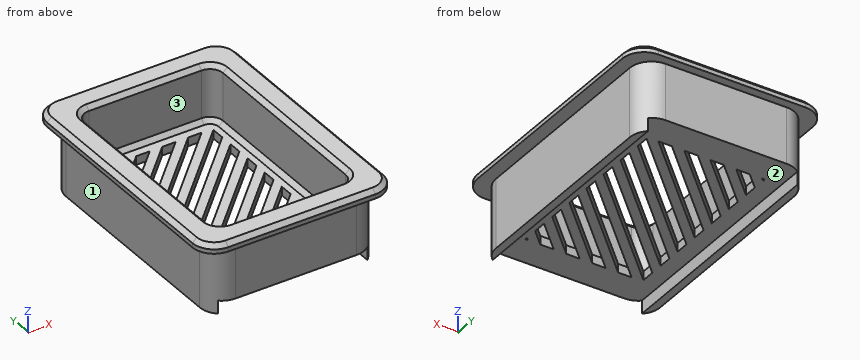
```python
from build123d import *

# Parameters (mm, degrees)
F0_W      = 28
F0_H      = 44
F1_DEPTH  = 2
F3_DEPTH  = 2
F4_W      = 38
F4_H      = 57
F4_W_2    = 27
F4_H_2    = 43
F5_DEPTH  = 2
F6_W      = 1.75
F6_H      = 57
F7_DEPTH  = 3
F8_W      = 38
F8_H      = 57
F8_W_2    = 32
F8_H_2    = 49
F9_DEPTH  = 11
F10_W     = 44
F10_H     = 61
F10_W_2   = 32
F10_H_2   = 49
F11_DEPTH = 2
F12_R     = 5
F13_R     = 3
F14_SIZE  = 1


with BuildPart() as f1:
    # F0 (on Top) → F1 (new body)
    with BuildSketch(Plane.XY):
        with Locations((-14, 22)):
            Rectangle(F0_W, F0_H)
    extrude(amount=F1_DEPTH)

    # F2 (on face) → F3 (cut, through all)
    with BuildSketch(Plane.XY.offset(2)):
        Polygon((-28, 48.4443650814), (-1.0000491969, 75.4443158845), (0, 79.5556349186), (-29.5556349186, 50), align=None)
        Polygon((0, 79.5556349186), (-1.0000491969, 75.4443158845), (1.5556349186, 78), align=None)
        Polygon((-28, 42.4443650814), (-2.9286171114, 67.51574797), (-1.9285679145, 71.6270670041), (-29.5556349186, 44), align=None)
        Polygon((-1.9285679145, 71.6270670041), (-2.9286171114, 67.51574797), (1.5556349186, 72), (0, 73.5556349186), align=None)
        Polygon((-28, 36.4443650814), (-4.8571850259, 59.5871800555), (-3.857135829, 63.6984990896), (-29.5556349186, 38), align=None)
        Polygon((-3.857135829, 63.6984990896), (-4.8571850259, 59.5871800555), (1.5556349186, 66), (0, 67.5556349186), align=None)
        Polygon((-28, 30.4443650814), (-6.7857529404, 51.658612141), (-5.7857037435, 55.7699311751), (-29.5556349186, 32), align=None)
        Polygon((-5.7857037435, 55.7699311751), (-6.7857529404, 51.658612141), (1.5556349186, 60), (0, 61.5556349186), align=None)
        Polygon((-28, 24.4443650814), (-8.7143208549, 43.7300442265), (-7.714271658, 47.8413632606), (-29.5556349186, 26), align=None)
        Polygon((-7.714271658, 47.8413632606), (-8.7143208549, 43.7300442265), (1.5556349186, 54), (0, 55.5556349186), align=None)
        Polygon((-28, 18.4443650814), (-10.6428887694, 35.8014763119), (-9.6428395725, 39.9127953461), (-29.5556349186, 20), align=None)
        Polygon((-9.6428395725, 39.9127953461), (-10.6428887694, 35.8014763119), (1.5556349186, 48), (0, 49.5556349186), align=None)
        Polygon((-28, 12.4443650814), (-12.5714566839, 27.8729083974), (-11.571407487, 31.9842274316), (-29.5556349186, 14), align=None)
        Polygon((-11.571407487, 31.9842274316), (-12.5714566839, 27.8729083974), (1.5556349186, 42), (0, 43.5556349186), align=None)
        Polygon((-28, 6.4443650814), (-14.5000245985, 19.9443404829), (-13.4999754015, 24.0556595171), (-29.5556349186, 8), align=None)
        Polygon((-13.4999754015, 24.0556595171), (-14.5000245985, 19.9443404829), (1.5556349186, 36), (0, 37.5556349186), align=None)
        Polygon((-28, 0.4443650814), (-16.428592513, 12.0157725684), (-15.4285433161, 16.1270916026), (-29.5556349186, 2), align=None)
        Polygon((-15.4285433161, 16.1270916026), (-16.428592513, 12.0157725684), (1.5556349186, 30), (0, 31.5556349186), align=None)
        Polygon((-28, -5.5556349186), (-18.3571604275, 4.0872046539), (-17.3571112306, 8.1985236881), (-29.5556349186, -4), align=None)
        Polygon((-17.3571112306, 8.1985236881), (-18.3571604275, 4.0872046539), (1.5556349186, 24), (0, 25.5556349186), align=None)
        Polygon((-28, -11.5556349186), (-20.285728342, -3.8413632606), (-19.2856791451, 0.2699557735), (-29.5556349186, -10), align=None)
        Polygon((-19.2856791451, 0.2699557735), (-20.285728342, -3.8413632606), (1.5556349186, 18), (0, 19.5556349186), align=None)
        Polygon((-28, -17.5556349186), (-22.2142962565, -11.7699311751), (-21.2142470596, -7.658612141), (-29.5556349186, -16), align=None)
        Polygon((-21.2142470596, -7.658612141), (-22.2142962565, -11.7699311751), (1.5556349186, 12), (0, 13.5556349186), align=None)
        Polygon((-28, -23.5556349186), (-24.142864171, -19.6984990896), (-23.1428149741, -15.5871800555), (-29.5556349186, -22), align=None)
        Polygon((-23.1428149741, -15.5871800555), (-24.142864171, -19.6984990896), (1.5556349186, 6), (0, 7.5556349186), align=None)
        Polygon((-28, -29.5556349186), (-26.0714320855, -27.6270670041), (-25.0713828886, -23.51574797), (-29.5556349186, -28), align=None)
        Polygon((-25.0713828886, -23.51574797), (-26.0714320855, -27.6270670041), (1.5556349186, 0), (0, 1.5556349186), align=None)
        Polygon((-26.9999508031, -31.4443158845), (-29.5556349186, -34), (-28, -35.5556349186), align=None)
        Polygon((0, -4.4443650814), (-26.9999508031, -31.4443158845), (-28, -35.5556349186), (1.5556349186, -6), align=None)
    extrude(amount=-F3_DEPTH, mode=Mode.SUBTRACT)

    # F4 (on Top) → F5 (join)
    with BuildSketch(Plane.XY):
        with Locations((-14, 22)):
            Rectangle(F4_W, F4_H)
        with Locations((-14, 22)):
            Rectangle(F4_W_2, F4_H_2, mode=Mode.SUBTRACT)
    extrude(amount=F5_DEPTH)

    # F6 (on face) → F7 (join)
    with BuildSketch(Plane(origin=(0, 0, 0), x_dir=(1, 0, 0), z_dir=(0, 0, -1))):
        with Locations((-32.125, -22)):
            Rectangle(F6_W, F6_H)
        with Locations((4.125, -22)):
            Rectangle(F6_W, F6_H)
    extrude(amount=F7_DEPTH)

    # F8 (on face) → F9 (join)
    with BuildSketch(Plane.XY.offset(2)):
        with Locations((-14, 22)):
            Rectangle(F8_W, F8_H)
        with Locations((-14, 22)):
            Rectangle(F8_W_2, F8_H_2, mode=Mode.SUBTRACT)
    extrude(amount=F9_DEPTH)

    # F10 (on face) → F11 (join)
    with BuildSketch(Plane.XY.offset(13)):
        with Locations((-14, 22)):
            Rectangle(F10_W, F10_H)
        with Locations((-14, 22)):
            Rectangle(F10_W_2, F10_H_2, mode=Mode.SUBTRACT)
    extrude(amount=F11_DEPTH)

    # F12
    f12_edges = [f1.edges().sort_by_distance(p)[0] for p in [
        (8, -8.5, 14),
        (5, -6.5, 5),
        (-33, -6.5, 5),
        (-36, -8.5, 14),
        (-36, 52.5, 14),
        (-33, 50.5, 5),
        (8, 52.5, 14),
        (5, 50.5, 5),
    ]]
    fillet(f12_edges, radius=F12_R)

    # F13
    f13_edges = [f1.edges().sort_by_distance(p)[0] for p in [
        (-30, 46.5, 8.5),
        (-30, -2.5, 8.5),
        (2, 46.5, 8.5),
        (2, -2.5, 8.5),
    ]]
    fillet(f13_edges, radius=F13_R)

    # F14
    f14_edges = [f1.edges().sort_by_distance(p)[0] for p in [
        (-14, 46.5, 2),
        (-14, 46.5, 15),
        (-36, 22, 15),
    ]]
    chamfer(f14_edges, length=F14_SIZE)


solid = f1.part
```
Input: part model. Units: mm. Frame: model coordinates. Face numbers are marked on the shaded views. A direction names the side the tool comes from. Give positions to 0.01 mm unless a question says otherwise; leave off trailing zeros. Order: outer loops, then holes, each group sorted by start corner. A loop starts at its lowest first (then second) coordinate and runs counter-clockwise, first axis right, second up. Notation, with made-up numbers: (46.5, 1) - (61.5, 1) arc R26 ccw to (61.5, 17) - close; hole circle Ø3 at (55, 38). An arc over 180 degrees is marked (long way). Use a Markdown table: item, result.
(1) Pin query (flat end, axial travel): pin 1 (5 mm diameter, centred on y = 23.5, z = 6, fed in from +X); pin 2 (10.5 mm diameter, centred on x = -13, z = 9, fed in from -Y); pin 3 (1 mm diameter, centred on x = -11.5, z = 1, fed in from -Y); pin 4 (3 mm diameter, centred on y = 39, z = 3.5, fed in from -X). Return the tip coordinate at first contact, or that it passes through.
Computed values:
| item | result |
|---|---|
| pin 1 | stops at x = 5 |
| pin 2 | stops at y = -8.5 |
| pin 3 | stops at y = -6.5 |
| pin 4 | stops at x = -33 |
(2) Section query B-B (z = 1). State how many separate pieces and enclosed holes the cut face has, then the cut area to 3 significant figures.
Computed values:
| item | result |
|---|---|
| separate pieces | 1 |
| enclosed holes | 13 |
| area | 1,540 mm2 |
(3) Section query A-A (z = 8). Output: boundary loops of the cut face in (x, y).
Computed values:
| item | result |
|---|---|
| outline | (-33, -1.5) arc R5 ccw to (-28, -6.5) - (0, -6.5) arc R5 ccw to (5, -1.5) - (5, 45.5) arc R5 ccw to (0, 50.5) - (-28, 50.5) arc R5 ccw to (-33, 45.5) - close; hole (-30, 0.5) arc R3 ccw to (-27, -2.5) - (-1, -2.5) arc R3 ccw to (2, 0.5) - (2, 43.5) arc R3 ccw to (-1, 46.5) - (-27, 46.5) arc R3 ccw to (-30, 43.5) - close |
(4) Access query for the marked faces 1, 2 and 3. Directions: +Z, -Z, +X, -X, +Y, -Y. A direction counts if a zero-diameter tool reaches every point of the face in a straight line with its end or side. Return the directions, or none.
Computed values:
| item | result |
|---|---|
| face 1 | -Z, -X, +Y, -Y |
| face 2 | -Z, +Y, -Y |
| face 3 | +Z |
(5) Line query: line 1 (X direction, y = 24, z = 12.5); line 2 (Y direction, x = -13, z = 4.75); line 3 (Z direction, x = -4, y = 44). Output: solid intervals per line, ascending. Write a range as from..to.
Computed values:
| item | result |
|---|---|
| line 1 | x = -33..-30, 2..5 |
| line 2 | y = -6.5..-2.5, 46.5..50.5 |
| line 3 | z = 0..2 |
